Part model, mm, in its own coordinate system. Give positions to 0.01 mm unless a question says otherwise; leave off trailing zeros. Write each loop counter-clockwise with the first axis right and the second up, starting at its lowest first coordinate (ties: lowest second). Pieces come first, ordered by that corner, then holes. Notation, with made-up numbers: M -27.5,73 L 15.5,73 A27 cw 15.5,95 Z; hole C 23.25,-25.5 d1. An arc over 180 degrees is marked long. Use a Markdown table: item, result.
```python
from build123d import *

# Parameters (mm, degrees)
BOSS_EXTRUDE1_DEPTH      = 115
BOSS_EXTRUDE1_DEPTH_BACK = 10
CUT_EXTRUDE1_DEPTH       = 10
SKETCH4_W                = 10.6
SKETCH4_H                = 62.2
CUT_EXTRUDE2_DEPTH       = 708.343268859


with BuildPart() as part:
    # Sketch2 → Boss-Extrude1 (new, two sides: drawn at the far end of the back side and taken through both)
    with BuildSketch(Plane.XY.offset(-BOSS_EXTRUDE1_DEPTH_BACK)):
        Polygon((321.928932188, 0), (329, 7.071067812), (-321.928932188, 658), (-329, 650.928932188), align=None)
    extrude(amount=BOSS_EXTRUDE1_DEPTH + BOSS_EXTRUDE1_DEPTH_BACK)

    # Sketch3 → Cut-Extrude1 (cut)
    with BuildSketch(Plane(origin=(160.964466094, 160.964466094, 0), x_dir=(-0.7071067811865476, 0.7071067811865476, 0), z_dir=(-0.7071067811865476, -0.7071067811865476, 0))):
        Polygon((-227.63813101, -115), (182.63813101, -115), (-227.63813101, 0), align=None)
        Polygon((692.914393031, -115), (282.63813101, -115), (692.914393031, 0), align=None)
    extrude(amount=-CUT_EXTRUDE1_DEPTH, mode=Mode.SUBTRACT)

    # Sketch4 → Cut-Extrude2 (cut, through all)
    with BuildSketch(Plane(origin=(160.964466094, 160.964466094, 0), x_dir=(-0.7071067811865476, 0.7071067811865476, 0), z_dir=(-0.7071067811865476, -0.7071067811865476, 0))):
        with Locations((232.63813101, -83.9)):
            Rectangle(SKETCH4_W, SKETCH4_H)
    extrude(amount=-CUT_EXTRUDE2_DEPTH, mode=Mode.SUBTRACT)


solid = part.part
```
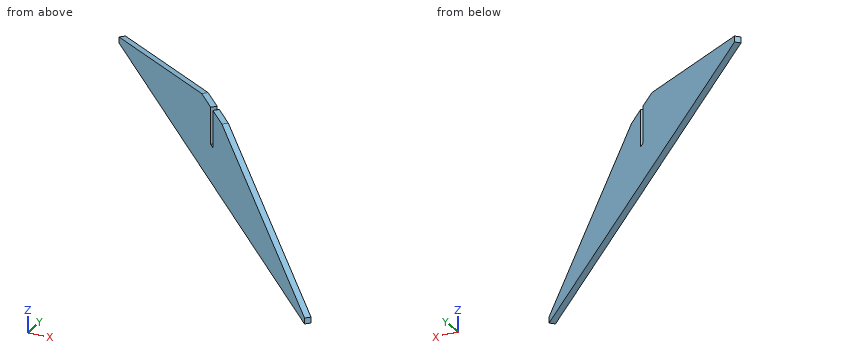
1. Cut at A-A, the plane z = 73. Give the cut face in (x, y).
Findings below:
| item | result |
|---|---|
| outline | M -144.84,466.77 L -7.28,329.21 L -0.21,336.28 L -137.77,473.84 Z; M 0.21,321.72 L 137.77,184.16 L 144.84,191.23 L 7.28,328.79 Z |
2. Cut at B-B, the plane y = 168.5. Give the cut face in (x, z), then the cut area to 3 significant figures.
Findings below:
| item | result |
|---|---|
| outline | M 153.43,-10 L 167.57,-10 L 167.57,63.99 L 153.43,66.79 Z |
| area | 1,070 mm2 |
3. Drill centre lines: L1, parallel to Y at x = 6.5, z = 93; L2, parallel to X at y = 398, z = 85.5; L3, parallel to X at y = 486, z = 39. Where is each one in solid material? Low to high.
Findings below:
| item | result |
|---|---|
| L1 | 315.43 to 328 |
| L2 | -76.07 to -61.93 |
| L3 | -164.07 to -149.93 |
4. Cut at C-C, the plane x = 107. Give the cut face in (y, z).
Findings below:
| item | result |
|---|---|
| outline | M 214.93,-10 L 229.07,-10 L 229.07,88 L 214.93,85.2 Z |
5. Drop flat-ended pins along their axis: P1, Ø1, axis at x = -115, z = 28, coming from the -Y side; P2, Ø12, axis at x = 69.5, z = 22, coming from the +Y side; P3, Ø6, axis at x = 206, z = 27.5, coming from the +Y side. Give the stop position or say it passes through.
Findings below:
| item | result |
|---|---|
| P1 | y = 436.43 |
| P2 | y = 272.57 |
| P3 | y = 133.07 |
